from build123d import *

# Parameters (mm, degrees)
CYLINDER_R            = 12
CYLINDER_DEPTH        = 2
SKETCH_R              = 1.5
POCKET_DEPTH          = 5
POLARPATTERN_COUNT    = 3
REVOLUTION_ANGLE      = 360
BOX_W                 = 12
BOX_H                 = 11
BOX_DEPTH             = 11
BOX_MIRRORED_2_W      = 12
BOX_MIRRORED_2_H      = 11
BOX_MIRRORED_2_DEPTH  = 11
POLARPATTERN001_COUNT = 3


with BuildPart() as part:
    # Cylinder → Cylinder (join)
    with BuildSketch(Plane.XY):
        Circle(CYLINDER_R)
    extrude(amount=CYLINDER_DEPTH)

    # Sketch → Pocket (cut)
    with BuildSketch(Plane.XY):
        with Locations((0, 8.9)):
            Circle(SKETCH_R)
    pocket = extrude(amount=POCKET_DEPTH, mode=Mode.SUBTRACT)

    # PolarPattern: Pocket ×3 about axis
    polarpattern_axis = Axis((0, 0, 0), (0, 0, 1))
    for i in range(1, POLARPATTERN_COUNT):
        add(pocket.rotate(polarpattern_axis, i * 360 / POLARPATTERN_COUNT), mode=Mode.SUBTRACT)

    # Sketch001 → Revolution (revolve, symmetric)
    with BuildSketch(Plane.YZ) as revolution_sk:
        with BuildLine():
            Line((-12, 2), (-3, 2))
            Line((-3, 2), (-3, 10))
            ThreePointArc((-3, 10), (-8.5, 7.125), (-12, 2))
        make_face()
    revolve(axis=Axis((0, 0, 0), (0, 0, 1)), revolution_arc=REVOLUTION_ANGLE / 2)
    revolve(revolution_sk.sketch, axis=Axis((0, 0, 0), (0, 0, -1)), revolution_arc=REVOLUTION_ANGLE / 2)

    # Box → Box (cut)
    with BuildSketch(Plane(origin=(2.5, -13, 2), x_dir=(0, 1, 0), z_dir=(1, 0, 0))):
        with Locations((6, 5.5)):
            Rectangle(BOX_W, BOX_H)
    box = extrude(amount=BOX_DEPTH, mode=Mode.SUBTRACT)

    # Box Mirrored 2 → Box Mirrored 2 (cut)
    with BuildSketch(Plane(origin=(-2.5, -13, 2), x_dir=(0, 1, 0), z_dir=(1, 0, 0))):
        with Locations((6, 5.5)):
            Rectangle(BOX_MIRRORED_2_W, BOX_MIRRORED_2_H)
    box_mirrored_2 = extrude(amount=-BOX_MIRRORED_2_DEPTH, mode=Mode.SUBTRACT)

    # PolarPattern001: Box, Box Mirrored 2 ×3 about axis
    polarpattern001_axis = Axis((0, 0, 0), (0, 0, 1))
    for i in range(1, POLARPATTERN001_COUNT):
        add(box.rotate(polarpattern001_axis, i * 360 / POLARPATTERN001_COUNT), mode=Mode.SUBTRACT)
        add(box_mirrored_2.rotate(polarpattern001_axis, i * 360 / POLARPATTERN001_COUNT), mode=Mode.SUBTRACT)


solid = part.part
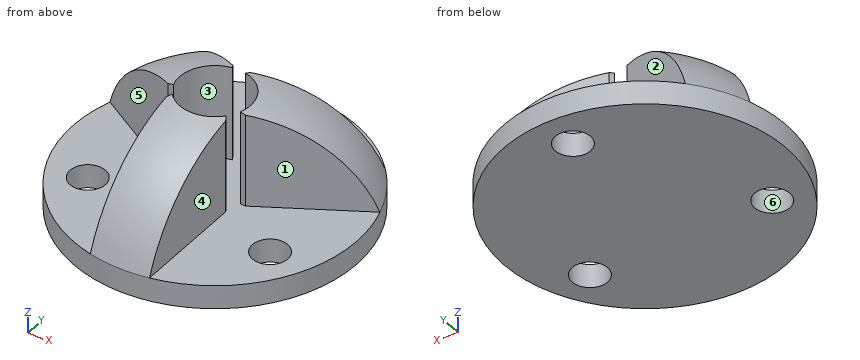
Part model, mm, in its own coordinate system. Face numbers are marked on the shaded views. A direction names the side the tool comes from. Coordinates: 2 decimals unless noted, no trailing zeros. Loops run counter-clockwise (first coordinate to the right, second up) from the corner with the lowest first, then second, coordinate; pieces in that order, holes last. Notation, with made-up numbers: M 22,-14.75 L 48,-14.75 A27 ccw 48,2.25 Z; hole C -5,82 d7. An arc over 180 degrees is marked long. Use a Markdown table: item, result. Add a question column.
Q1. Pin check, flat tips, straight feed: P1, Ø3, axis at x = -5.5, z = 4, coming from the +Y side; P2, Ø1.5, axis at x = -2, y = 7.5, coming from the +Z side; P3, Ø3, axis at x = 4.5, y = 1.5, coming from the +Z side; P4, Ø1.8, axis at x = 0, y = 8.9, coming from the -Z side. Stop position of each tip, or through.
Q2. Which spindle directions (+Z, -Z, +X, -X, +Y, -Y) get a long thin tool onto all of the face, cutting with end or side? Do the marked faces 1, 2 and 3. Say none if no direction does.
Q3. Cut at D-D (y = -4.45). Write the cut outline in (x, z), and give its area (3 significant figures).
Q4. Cut at B-B (y = 8.9). Write the cut outline in (x, z).
Q5. Mould opens along Y. For the marked faces 4, 5 and 6 say: +Y half, -Y half, draft (parallel to the pull), parting line (faces both ways), or undercut.
Q6. Probe L1, parallel to Z at x = -6.25, y = 8.5; L2, parallel to X at y = 0, z = 6; L3, parallel to X at y = 8.9, z = 1.65. List the from-to ranges inside material, lowest first.
Q7. Cut at A-A (x = 0). Write the cut outline in (y, z), and give its area (3 significant figures).
Q8. Cut at C-C (z = 7.75). Write the cut outline in (x, y), and give its area (3 significant figures).
Worked out:
| question | item | result |
|---|---|---|
| 1 | P1 | stops at y = 6.93 |
| 1 | P2 | stops at z = 2 |
| 1 | P3 | stops at z = 9.94 |
| 1 | P4 | passes through |
| 2 | face 1 | +Z, +X, -Y |
| 2 | face 2 | +Z, +Y |
| 2 | face 3 | +Z |
| 3 | outline | M -11.14,0 L -9.21,0 L -9.21,2 L -11.14,2 Z; M -6.21,0 L 6.21,0 L 6.21,2 L 2.5,2 L 2.5,9.29 A12 ccw -2.5,9.29 L -2.5,2 L -6.21,2 Z; M 9.21,0 L 11.14,0 L 11.14,2 L 9.21,2 Z |
| 3 | area | 69.9 mm2 |
| 4 | outline | M -8.05,0 L -1.5,0 L -1.5,2 L -8.05,2 Z; M 1.5,0 L 8.05,0 L 8.05,2 L 1.5,2 Z |
| 5 | face 4 | draft |
| 5 | face 5 | -Y half |
| 5 | face 6 | undercut |
| 6 | L1 | z = 0 to 2 |
| 6 | L2 | x = -5 to -3, 3 to 5 |
| 6 | L3 | x = -8.05 to -1.5, 1.5 to 8.05 |
| 7 | outline | M -12,0 L 7.4,0 L 7.4,2 L -3,2 L -3,10 A12.79 ccw -12,2 Z; M 10.4,0 L 12,0 L 12,2 L 10.4,2 Z |
| 7 | area | 90.2 mm2 |
| 8 | outline | M -7.59,1.5 L -3.27,-1 L -2.83,-1 A3 cw -0.55,2.95 L -0.77,3.33 L -5.09,5.83 A7.74 ccw Z; M -2.5,-7.33 A7.74 ccw 2.5,-7.33 L 2.5,-2.33 L 2.28,-1.95 A3 cw -2.28,-1.95 L -2.5,-2.33 Z; M 0.55,2.95 A3 cw 2.83,-1 L 3.27,-1 L 7.59,1.5 A7.74 ccw 5.09,5.83 L 0.77,3.33 Z |
| 8 | area | 74.6 mm2 |
